```python
from build123d import *

# Parameters (mm, degrees)
SKETCH1_W           = 254
SKETCH1_H           = 152.4
SKETCH1_W_2         = 6.35
SKETCH1_H_2         = 139.7
SKETCH1_W_3         = 3.175
SKETCH1_W_4         = 100.0125
SKETCH1_H_3         = 6.34492
BOSS_EXTRUDE1_DEPTH = 6.35


with BuildPart() as part:
    # Sketch1 → Boss-Extrude1 (new body)
    with BuildSketch(Plane(origin=(0, 0, 0), x_dir=(1, 0, 0), z_dir=(0, 1, 0))):
        Rectangle(SKETCH1_W, SKETCH1_H)
        with Locations((117.475, 0)):
            Rectangle(SKETCH1_W_2, SKETCH1_H_2, mode=Mode.SUBTRACT)
        Rectangle(SKETCH1_W_3, SKETCH1_H_2, mode=Mode.SUBTRACT)
        with Locations((-117.475, 0)):
            Rectangle(SKETCH1_W_2, SKETCH1_H_2, mode=Mode.SUBTRACT)
        with Locations((-57.94375, 66.67754)):
            Rectangle(SKETCH1_W_4, SKETCH1_H_3, mode=Mode.SUBTRACT)
        with Locations((57.94375, -66.68262)):
            Rectangle(SKETCH1_W_4, SKETCH1_H_3, mode=Mode.SUBTRACT)
        with Locations((57.94375, 66.67754)):
            Rectangle(SKETCH1_W_4, SKETCH1_H_3, mode=Mode.SUBTRACT)
        with Locations((-57.94375, -66.67754)):
            Rectangle(SKETCH1_W_4, SKETCH1_H_3, mode=Mode.SUBTRACT)
    extrude(amount=BOSS_EXTRUDE1_DEPTH)


solid = part.part
```
Design review of the part built by this model. Coordinates are the model's own, in mm. Give positions to 0.01 mm unless a question says otherwise; leave off trailing zeros. Order: outer loops, then holes, each group sorted by start corner. A loop starts at its lowest first (then second) coordinate and runs counter-clockwise, first axis right, second up. Notation, with made-up numbers: (73.5, 12.25) -> (88.5, 12.25) arc R22 ccw to (88.5, 26.25) -> close; hole circle Ø5 at (13, 52). An arc over 180 degrees is marked (long way). Write item = value, one per line. Start each with the question number.
(1) Mouldability with a two-part tool opening along Z and no side actions: class faces 1 (the face through (127, 3, 1)), 2 (the face through (1.588, 3, 1)) as +Z half, -Z half, draft (parallel to the pull), parting line (faces both ways), or undercut.
(2) To check wall thickness, follow line 1 along X through (y, z) = (2.75, -55); line 2 along X through (y, z) = (5.5, 67); line 3 along Z through (x, y) = (-90, 1.5). State the ranges of each line that lie inside material, in increasing order.
(3) We need section A-A on z = -56.5. Write out the cut boundary in (x, y).
(4) We need section B-B on x = 80. Write out the cut boundary in (y, z), plus the area to 3 significant figures.
(5) We need section C-C on y = 1.25. State how many separate pieces and enclosed holes the cut face has, plus the area to 3 significant figures.
Numbers:
q1.face_1 = draft
q1.face_2 = undercut
q2.line_1 = -127 to -120.65, -114.3 to -1.59, 1.59 to 114.3, 120.65 to 127
q2.line_2 = -127 to -120.65, -114.3 to -107.95, -7.94 to -1.59, 1.59 to 7.94, 107.95 to 114.3, 120.65 to 127
q2.line_3 = -76.2 to -69.85, -63.51 to 63.51, 69.85 to 76.2
q3.outline = (-127, 0) -> (-120.65, 0) -> (-120.65, 6.35) -> (-127, 6.35) -> close; (-114.3, 0) -> (-1.59, 0) -> (-1.59, 6.35) -> (-114.3, 6.35) -> close; (1.59, 0) -> (114.3, 0) -> (114.3, 6.35) -> (1.59, 6.35) -> close; (120.65, 0) -> (127, 0) -> (127, 6.35) -> (120.65, 6.35) -> close
q4.outline = (0, -76.2) -> (6.35, -76.2) -> (6.35, -69.85) -> (0, -69.85) -> close; (0, -63.51) -> (6.35, -63.51) -> (6.35, 63.51) -> (0, 63.51) -> close; (0, 69.86) -> (6.35, 69.86) -> (6.35, 76.2) -> (0, 76.2) -> close
q4.area = 887 mm^2
q5.separate_pieces = 1
q5.enclosed_holes = 7
q5.area = 34,000 mm^2
